Work out the finished part from the listing and answer in its coordinate system (mm). A direction names the side the tool comes from. Round coordinates to 2 decimals unless told otherwise and drop trailing zeros. Write each loop counter-clockwise with the first axis right and the second up, starting at its lowest first coordinate (ties: lowest second). Pieces come first, ordered by that corner, then holes. Notation, with made-up numbers: (21.25, 3) -> (54.25, 3) arc R32 cw to (54.25, 35) -> close; hole circle Ø7 at (65.5, 67). An arc over 180 degrees is marked (long way). Answer as a JSON object with one key per item and string values. Group by question number.
from build123d import *

# Parameters (mm, degrees)
BOSS_EXTRUDE1_DEPTH      = 60
CUT_EXTRUDE1_DEPTH       = 26
BOSS_EXTRUDE2_DEPTH      = 34
BOSS_EXTRUDE2_DEPTH_BACK = 9
SKETCH4_R                = 5
CUT_EXTRUDE2_DEPTH       = 117
CUT_EXTRUDE3_DEPTH       = 31
BOSS_EXTRUDE3_START      = -11.652052
SKETCH7_R                = 21.124192
SKETCH7_R_2              = 13
BOSS_EXTRUDE3_DEPTH      = 22.652052
FILLET1_R                = 10


with BuildPart() as part:
    # Sketch2 → Boss-Extrude1 (new body)
    with BuildSketch(Plane.XY):
        Polygon((-14.104352, 47.779255), (-57.46381, 47.779255), (-57.46381, -13.919632), (-13.887058, -13.919632), (-13.887058, -23.919632), (-69.115862, -23.919632), (-69.115862, 57.003505), (-14.104352, 57.003505), align=None)
    extrude(amount=BOSS_EXTRUDE1_DEPTH)

    # Sketch3 → Cut-Extrude1 (cut)
    with BuildSketch(Plane(origin=(-14.104352, 0, 0), x_dir=(0, 0, -1), z_dir=(1, 0, 0))):
        Polygon((-43.271654, -23.143882), (-43.271654, 57.003505), (-16.728346, 57.003505), (-16.728346, -23.143882), (-16.728346, -35.223541), (-43.271654, -35.223541), align=None)
    extrude(amount=-CUT_EXTRUDE1_DEPTH, mode=Mode.SUBTRACT)

    # Sketch4 → Boss-Extrude2 (add, two sides: drawn at the far end of the back side and taken through both)
    with BuildSketch(Plane.XY.offset(16.728346).offset(-BOSS_EXTRUDE2_DEPTH_BACK)):
        with Locations(Location((-14.104352, 52.39138, 0), (0, 0, 247.283219))):
            Circle(SKETCH4_R)
        with Locations((-13.887058, -18.919632)):
            Circle(SKETCH4_R)
    extrude(amount=BOSS_EXTRUDE2_DEPTH + BOSS_EXTRUDE2_DEPTH_BACK)

    # Sketch5 → Cut-Extrude2 (cut)
    with BuildSketch(Plane(origin=(0, 57.003505, 0), x_dir=(1, 0, 0), z_dir=(0, 1, 0))):
        Polygon((-14.104352, -7.728346), (-16.035233, -7.728346), (-69.115862, -15.56073), (-69.115862, 0), (-12.569793, 0), align=None)
        Polygon((-69.115862, -44.179694), (-16.035233, -50.728346), (-13.887058, -50.728346), (-13.887058, -60), (-69.115862, -60), align=None)
    extrude(amount=-CUT_EXTRUDE2_DEPTH, mode=Mode.SUBTRACT)

    # Sketch6 → Cut-Extrude3 (cut)
    with BuildSketch(Plane.ZY.offset(69.115862)):
        with BuildLine():
            ThreePointArc((42.870212, 16.541936), (29.870212, 29.541936), (16.870212, 16.541936))
            Line((16.870212, 16.541936), (42.870212, 16.541936))
        make_face()
        with BuildLine():
            Line((42.870212, 16.541936), (16.870212, 16.541936))
            ThreePointArc((16.870212, 16.541936), (29.870212, 3.541936), (42.870212, 16.541936))
        make_face()
    extrude(amount=-CUT_EXTRUDE3_DEPTH, mode=Mode.SUBTRACT)

    # Sketch7 → Boss-Extrude3 (add)
    with BuildSketch(Plane.ZY.offset(69.115862).offset(BOSS_EXTRUDE3_START)):
        with Locations((29.870212, 16.541936)):
            Circle(SKETCH7_R)
        with Locations((29.870212, 16.541936)):
            Circle(SKETCH7_R_2, mode=Mode.SUBTRACT)
    extrude(amount=BOSS_EXTRUDE3_DEPTH)

    # Fillet1
    fillet1_edges = [part.edges().sort_by_distance(p)[0] for p in [
        (-57.46381, -13.919632, 29.729312),
        (-57.46381, 47.779255, 29.729312),
        (-69.115862, 57.003505, 29.870212),
        (-69.115862, -23.919632, 29.870212),
    ]]
    fillet(fillet1_edges, radius=FILLET1_R)


solid = part.part
1) Each of these flat-tipped pins is pushed along its axis until it touches: P1, Ø1.5, axis at y = 32.5, z = 31, coming from the +X side; P2, Ø3, axis at y = -10, z = 40.5, coming from the -X side; P3, Ø2, axis at x = -14, y = -19, coming from the +Z side; P4, Ø21, axis at y = 16.54, z = 29.87, coming from the +X side. Where does it stop, or does it pass through?
2) A tool of negligible diameter and unlimited length cuts with its end or side. For faces 4 (the face through (-71.148, 17.471, 8.766)), 5 (the face through (-40.104, -19, 30)), 6 (the face through (-48.1, -16.32, 12.46)), 7 (the face through (-54.457, 44.928, 29.85)), 8 (the face through (-48.84, 49.86, 46.68)), from which of +Z, -Z, +X, -X, +Y, -Y can it reach the whole face along a straight path? Write none if from no direction.
3) Straight lines are drawn through the part: L1, parallel to X at y = -4.5, z = 25; L2, parallel to X at y = 33, z = 18; L3, parallel to Y at x = -70.5, z = 20. For each, find the intervals that lie inside material, in ascending order.
4) A cutting plane is placed at D-D on x = -42.5. Determine the outline of the cut face in (y, z).
5) A cutting plane is placed at A-A on x = -29.5. Determine the outline of the cut face in (y, z), plus the area to 3 significant figures.
6) A cutting plane is placed at B-B on y = 15. Determine the outline of the cut face in (x, z).
7) A cutting plane is placed at C-C on z = 28. State how many separate pieces and enclosed holes the cut face has, plus the area to 3 significant figures.
8) For a pull along Y with two mould halves and no side action, classify faces 1 (the face through (-54.457, -11.068, 29.85)), 2 (the face through (-43, 57.004, 29)), 3 (the face through (-48.84, -16.41, 46.68)) as released by +Y, released by -Y, zero draft, split by the parting line, or undercut.
Established:
{
 "1": {"P1": "stops at x = -57.46", "P2": "stops at x = -69.12", "P3": "stops at z = 50.73", "P4": "passes through"},
 "2": {"face 4": "-X", "face 5": "+Y, -Y", "face 6": "-Z, -X, -Y", "face 7": "+Z, -Z", "face 8": "+Z, -X, +Y"},
 "3": {"L1": "x = -69.12 to -57.45", "L2": "x = -80.12 to -57.46", "L3": "y = -2.13 to 8.08, 25 to 35.22"},
 "4": {"outline": "(-23.92, 11.63) -> (-13.92, 11.63) -> (-13.92, 47.46) -> (-23.92, 47.46) -> close; (47.78, 11.63) -> (57, 11.63) -> (57, 47.46) -> (47.78, 47.46) -> close"},
 "5": {"outline": "(-23.92, 9.72) -> (-13.92, 9.72) -> (-13.92, 16.73) -> (-23.92, 16.73) -> close; (-23.92, 43.27) -> (-13.92, 43.27) -> (-13.92, 49.07) -> (-23.92, 49.07) -> close; (47.78, 9.72) -> (57, 9.72) -> (57, 16.73) -> (47.78, 16.73) -> close; (47.78, 43.27) -> (57, 43.27) -> (57, 49.07) -> (47.78, 49.07) -> close", "area": "246 mm²"},
 "6": {"outline": "(-80.12, 8.8) -> (-57.46, 8.8) -> (-57.46, 16.96) -> (-80.12, 16.96) -> close; (-80.12, 42.78) -> (-57.46, 42.78) -> (-57.46, 50.94) -> (-80.12, 50.94) -> close"},
 "7": {"separate pieces": "4", "enclosed holes": "0", "area": "1,310 mm²"},
 "8": {"face 1": "undercut", "face 2": "released by +Y", "face 3": "zero draft"}
}
